Could you check a few things on this model? Use its own coordinates, in mm. A direction names the side the tool comes from. Coordinates: 2 decimals unless noted, no trailing zeros. Loops run counter-clockwise (first coordinate to the right, second up) from the corner with the lowest first, then second, coordinate; pieces in that order, holes last. Notation, with made-up numbers: (-7, -15.75) - (-3, -15.75) arc R32 cw to (-3, 11.25) - close; hole circle Ø9 at (-29, 23). An arc over 180 degrees is marked (long way). One line per question, with ' | ' between items. Start each with the question number.
1. Which directions (+Z, -Z, +X, -X, +Y, -Y) give clear straight access to the entire face, cutting with the end or side of a thin tool? Please do faces 1 (the flat face through (-14, -5.5, -14)), 2 (the flat face through (0, 3, 0)), 3 (the cylindrical face through (9.9, 11.2, 13.5)).
2. We'd pull the mould along X, two halves only. Please class faces 4 (the flat face through (19, 14.5, 0)), 5 (the cylindrical face through (-17.394, 11.218, 13.482)): pulls with the +X half, pulls with the -X half, needs draft (parallel to the pull), parting line crosses it, or undercut.
3. Please list where these lines run through material, in increasing order: L1, parallel to Z at x = 16, y = 9.5; L2, parallel to Y at x = 3, z = 15.5; L3, parallel to X at y = 7.7, z = 0. Write a range as [from, to].
4. I want a section at C-C, the plane y = 4. Write out the boundary of the cut face in (x, z).
5. I want a section at B-B, the plane y = 1. Write out the boundary of the cut face in (x, z).
6. I'm going to push flat-ended pins straight in: P1, Ø3.5, axis at x = -2.5, z = 3, coming from the -Y side; P2, Ø1.5, axis at y = 10.5, z = -10, coming from the +X side; P3, Ø1, axis at y = 4, z = 19, coming from the +X side; P4, Ø1, axis at y = -1, z = -7.5, coming from the +X side. Where does each tip first touch, or does it pass through?
7. I want a section at A-A, the plane y = 11.75. Write out the boundary of the cut face in (x, z).
from build123d import *

# Parameters (mm, degrees)
SKETCH1_R           = 26
BOSS_EXTRUDE1_DEPTH = 9
SKETCH2_R           = 6.1
CUT_EXTRUDE2_DEPTH  = 3
CUT_EXTRUDE5_START  = 9
SKETCH1_9_R         = 6.25
CUT_EXTRUDE5_DEPTH  = 3
SKETCH1_11_R        = 3.75
BOSS_EXTRUDE3_DEPTH = 5.5
BOSS_EXTRUDE4_START = 9
SKETCH1_12_R        = 3.75
BOSS_EXTRUDE4_DEPTH = 5.5
CHAMFER1_SIZE       = 1
FILLET1_R           = 2.5


with BuildPart() as part:
    # Sketch1 → Boss-Extrude1 (new body)
    with BuildSketch(Plane(origin=(0, 0, 0), x_dir=(1, 0, 0), z_dir=(0, 1, 0))):
        Circle(SKETCH1_R)
    extrude(amount=BOSS_EXTRUDE1_DEPTH)

    # Sketch2 → Cut-Extrude2 (cut)
    with BuildSketch(Plane.XZ):
        Circle(SKETCH2_R)
    extrude(amount=-CUT_EXTRUDE2_DEPTH, mode=Mode.SUBTRACT)

    # Sketch1<9> → Cut-Extrude5 (cut)
    with BuildSketch(Plane(origin=(0, 0, 0), x_dir=(1, 0, 0), z_dir=(0, 1, 0)).offset(CUT_EXTRUDE5_START)):
        Circle(SKETCH1_9_R)
    extrude(amount=-CUT_EXTRUDE5_DEPTH, mode=Mode.SUBTRACT)

    # Sketch1<11> → Boss-Extrude3 (add)
    with BuildSketch(Plane(origin=(0, 0, 0), x_dir=(1, 0, 0), z_dir=(0, 1, 0))):
        with Locations((-13.647160877, 13.647160877)):
            Circle(SKETCH1_11_R)
        with Locations((0, 19.3)):
            Circle(SKETCH1_11_R)
        with Locations((13.647160877, 13.647160877)):
            Circle(SKETCH1_11_R)
        with Locations((19.3, 0)):
            Circle(SKETCH1_11_R)
        with Locations((13.647160877, -13.647160877)):
            Circle(SKETCH1_11_R)
        with Locations((0, -19.3)):
            Circle(SKETCH1_11_R)
        with Locations((-13.647160877, -13.647160877)):
            Circle(SKETCH1_11_R)
        with Locations((-19.3, 0)):
            Circle(SKETCH1_11_R)
    extrude(amount=-BOSS_EXTRUDE3_DEPTH)

    # Sketch1<12> → Boss-Extrude4 (add)
    with BuildSketch(Plane(origin=(0, 0, 0), x_dir=(1, 0, 0), z_dir=(0, 1, 0)).offset(BOSS_EXTRUDE4_START)):
        with Locations((-13.647160877, 13.647160877)):
            Circle(SKETCH1_12_R)
        with Locations((0, 19.3)):
            Circle(SKETCH1_12_R)
        with Locations((13.647160877, 13.647160877)):
            Circle(SKETCH1_12_R)
        with Locations((19.3, 0)):
            Circle(SKETCH1_12_R)
        with Locations((13.647160877, -13.647160877)):
            Circle(SKETCH1_12_R)
        with Locations((0, -19.3)):
            Circle(SKETCH1_12_R)
        with Locations((-13.647160877, -13.647160877)):
            Circle(SKETCH1_12_R)
        with Locations((-19.3, 0)):
            Circle(SKETCH1_12_R)
    extrude(amount=BOSS_EXTRUDE4_DEPTH)

    # Chamfer1
    chamfer1_edges = [part.edges().sort_by_distance(p)[0] for p in [
        (-17.397160877, -5.5, -13.647160877),
        (-3.75, -5.5, -19.3),
        (9.897160877, -5.5, -13.647160877),
        (15.55, -5.5, 0),
        (9.897160877, -5.5, 13.647160877),
        (-3.75, -5.5, 19.3),
        (-17.397160877, -5.5, 13.647160877),
        (-23.05, -5.5, 0),
        (15.55, 14.5, 0),
        (9.897160877, 14.5, -13.647160877),
        (-3.75, 14.5, -19.3),
        (-17.397160877, 14.5, -13.647160877),
        (-3.75, 14.5, 19.3),
        (9.897160877, 14.5, 13.647160877),
        (-23.05, 14.5, 0),
        (-17.397160877, 14.5, 13.647160877),
    ]]
    chamfer(chamfer1_edges, length=CHAMFER1_SIZE)

    # Fillet1
    fillet1_edges = [part.edges().sort_by_distance(p)[0] for p in [
        (-26, 0, 0),
        (-26, 9, 0),
    ]]
    fillet(fillet1_edges, radius=FILLET1_R)


solid = part.part
Results are:
1) face 1: +Z, -Z, +X, -X, -Y | face 2: -Y | face 3: +Y
2) face 4: needs draft | face 5: undercut
3) L1: z = [-16.57, -10.73], [-1.78, 1.78], [10.73, 16.57] | L2: y = [0, 9] | L3: x = [-25.69, -6.25], [6.25, 25.69]
4) outline: circle Ø52 at (0, 0)
5) outline: circle Ø51 at (0, 0); hole circle Ø12.2 at (0, 0)
6) P1: stops at y = 3 | P2: stops at x = 16.03 | P3: stops at x = 18.27 | P4: passes through
7) outline: circle Ø7.5 at (-19.3, 0); circle Ø7.5 at (-13.65, -13.65); circle Ø7.5 at (-13.65, 13.65); circle Ø7.5 at (0, -19.3); circle Ø7.5 at (0, 19.3); circle Ø7.5 at (13.65, -13.65); circle Ø7.5 at (13.65, 13.65); circle Ø7.5 at (19.3, 0)
